Can you work these out from the model? Positions are in its coordinate system, mm. Face numbers are marked on the shaded views. A direction names the side the tool comes from. Round coordinates to 2 decimals unless told otherwise and drop trailing zeros. Loops run counter-clockwise (first coordinate to the right, second up) from the corner with the lowest first, then second, coordinate; pieces in that order, holes last. Notation, with made-up numbers: (-32.5, -38) -> (-18.5, -38) arc R24 ccw to (-18.5, -19) -> close; hole circle Ø11 at (88, 84.25). An arc over 180 degrees is marked (long way). Answer as a JSON object with one key per item and string values.
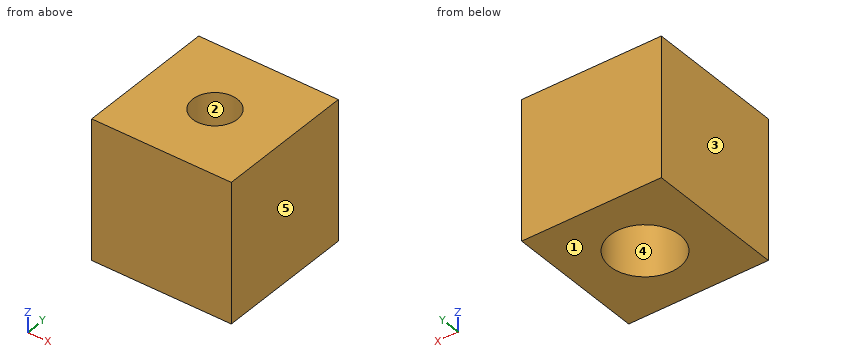
```python
from build123d import *

# Parameters (mm, degrees)
F0_W     = 100
F0_H     = 100
F1_DEPTH = 100
F2_D     = 32
F3_D     = 50
F3_DEPTH = 50
F3_TIP   = 15.0215154757


with BuildPart() as f1:
    # F0 (on Top) → F1 (new body)
    with BuildSketch(Plane.XY):
        Rectangle(F0_W, F0_H)
    extrude(amount=F1_DEPTH)

    # F2 (through all)
    with Locations(Plane(origin=(0, 0, 0), x_dir=(1, 0, 0), z_dir=(0, 0, -1))):
        with Locations((0, 0)):
            Hole(F2_D / 2)

    # F3
    with Locations(Plane(origin=(0, 0, 0), x_dir=(1, 0, 0), z_dir=(0, 0, -1))):
        with Locations((0, 0)):
            Hole(F3_D / 2, depth=F3_DEPTH)
            with Locations((0, 0, -(F3_DEPTH + F3_TIP / 2))):  # 118° drill point
                Cone(0, F3_D / 2, F3_TIP, mode=Mode.SUBTRACT)


solid = f1.part
```
Q1. I want a section at A-A, the plane y = 0. Write out the boundary of the cut face in (x, z).
Determined:
{"outline": "(-50, 0) -> (-25, 0) -> (-25, 50) -> (-16, 55.41) -> (-16, 100) -> (-50, 100) -> close; (16, 55.41) -> (25, 50) -> (25, 0) -> (50, 0) -> (50, 100) -> (16, 100) -> close"}
Q2. We'd pull the mould along X, two halves only. Please class the marked faces 1, 2 and 3: pulls with the +X half, pulls with the -X half, needs draft (parallel to the pull), parting line crosses it, or undercut.
Determined:
{"face 1": "needs draft", "face 2": "undercut", "face 3": "pulls with the -X half"}
Q3. On a 3-axis mill with a long thin cutter (end or side, diameter ignored), from which of +Z, -Z, +X, -X, +Y, -Y can I reach the whole of each face in a straight line? I mean the marked faces 4 and 5. Say none if no direction works.
Determined:
{"face 4": "-Z", "face 5": "+Z, -Z, +X, +Y, -Y"}
Q4. I want a section at D-D, the plane z = 93. Write out the boundary of the cut face in (x, y).
Determined:
{"outline": "(-50, -50) -> (50, -50) -> (50, 50) -> (-50, 50) -> close; hole circle Ø32 at (0, 0)"}
Q5. I want a section at C-C, the plane z = 15.5. Write out the boundary of the cut face in (x, y), then the cut area to 3 significant figures.
Determined:
{"outline": "(-50, -50) -> (50, -50) -> (50, 50) -> (-50, 50) -> close; hole circle Ø50 at (0, 0)", "area": "8,040 mm²"}
Q6. If I drill on L1, parallel to Y at x = 0, z = 31; L2, parallel to Y at x = 0, z = 86; L3, parallel to X at y = -11, z = 63.5, over which ranges is the centre line in solid material (lowest first)? Write a range as [from, to].
Determined:
{"L1": "[-50, -25], [25, 50]", "L2": "[-50, -16], [16, 50]", "L3": "[-50, -11.62], [11.62, 50]"}
